```python
from build123d import *

# Parameters (mm, degrees)
CHAMFER1_SIZE = 1
FILLET2_R     = 1


with BuildPart() as part:
    # Sketch1 → Revolve1 (revolve)
    with BuildSketch(Plane.XY, mode=Mode.PRIVATE) as revolve1_sk:
        Polygon((-5, 0), (-13, 0), (-13, 6.5), (-10, 6.5), (-10, 15.5), (-8.9, 15.5), (-8.9, 16.8), (-10, 16.8), (-10, 24), (-6, 24), (-6, 62.5), (-4.9, 62.5), (-4.9, 63.8), (-6, 63.8), (-6, 68), (0, 68), (0, 18), (-5, 18), align=None)
    revolve(revolve1_sk.sketch.rotate(Axis((0, 0, 0), (0, 1, 0)), 180), axis=Axis((0, 0, 0), (0, 1, 0)))

    # Chamfer1
    chamfer1_edges = [part.edges().sort_by_distance(p)[0] for p in [
        (-10, 24, 0),
        (-6, 68, 0),
        (-5, 0, 0),
        (-13, 0, 0),
        (-13, 6.5, 0),
    ]]
    chamfer(chamfer1_edges, length=CHAMFER1_SIZE)

    # Fillet2
    fillet2_edges = [part.edges().sort_by_distance(p)[0] for p in [
        (-6, 24, 0),
    ]]
    fillet(fillet2_edges, radius=FILLET2_R)


solid = part.part
```
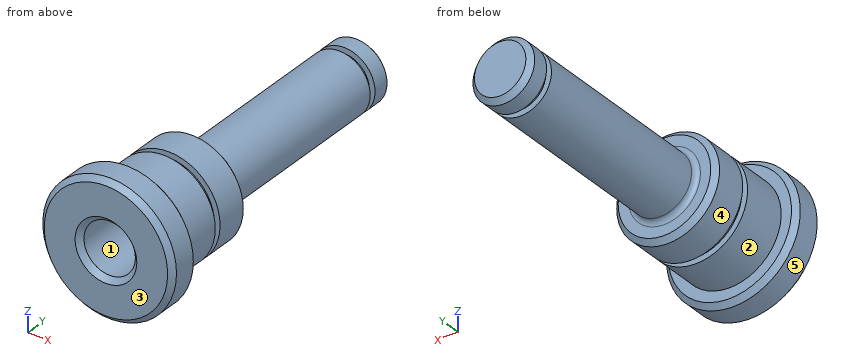
Geometry check sheet. Reference: the model listing, model coordinates, mm. Face numbers are marked on the shaded views. A direction names the side the tool comes from. Coordinates: 2 decimals unless noted, no trailing zeros. Order: outer loops, then holes, each group sorted by start corner. A loop starts at its lowest first (then second) coordinate and runs counter-clockwise, first axis right, second up.
Q1. Thickness scan on probe 1 along Z at (x, y) = (0, 11.75); probe 2 along Y at (x, z) = (7.75, 7.25); probe 3 along Y at (x, z) = (-8, -5). Record the ranges inside material, lowest first.
Reply:
probe 1: z = -10 to -5, 5 to 10
probe 2: y = 0 to 6.5
probe 3: y = 0 to 15.5, 16.8 to 23.57
Q2. Sectioned sample at B-B on y = 28.5. Record the cut outline in (x, z), and give its area (3 significant figures).
Reply:
outline: circle Ø12 at (0, 0)
area: 113 mm2
Q3. Depth check by flat-ended pin: pin 1 Ø1.5 at (x, y) = (-5.5, 54.5) entering from -Z; pin 2 Ø1.5 at (x, z) = (-4, 9) entering from +Y; pin 3 Ø10 at (y, z) = (43, 2.5) entering from +X. Enter the tip coordinate at first touch or a pass-through.
Reply:
pin 1: stops at z = -3.67
pin 2: stops at y = 23.9
pin 3: stops at x = 6
Q4. Sectioned sample at A-A on y = 8.5. Record the cut outline in (x, z), and give its area (3 significant figures).
Reply:
outline: circle Ø20 at (0, 0); hole circle Ø10 at (0, 0)
area: 236 mm2
Q5. Tool access check on the marked faces 4 and 5. Record the directions out of +Z, -Z, +X, -X, +Y, -Y that give a thin tool (end or side, any length) a straight path to the whole face; none if there is none.
Reply:
face 4: +Y
face 5: +Y, -Y
Q6. Draft check along Z on the marked faces 1, 2 and 3. Enter one of: released by +Z, released by -Z, zero draft, split by the parting line, or undercut.
Reply:
face 1: undercut
face 2: split by the parting line
face 3: zero draft
